from build123d import *

# Parameters (mm, degrees)
SKETCH1_W           = 31.5
SKETCH1_H           = 26
BOSS_EXTRUDE1_DEPTH = 33
SKETCH8_W           = 16
SKETCH8_H           = 20
BOSS_EXTRUDE2_DEPTH = 8
CUT_EXTRUDE1_START  = 10
CUT_EXTRUDE1_DEPTH  = 40.164116391
SKETCH3_R           = 2.85
CUT_EXTRUDE2_DEPTH  = 50.204293512
SKETCH6_R           = 6.25
CUT_EXTRUDE5_DEPTH  = 2
SKETCH4_R           = 2.35
CUT_EXTRUDE3_DEPTH  = 50.164116391
SKETCH5_R           = 6.5
CUT_EXTRUDE4_DEPTH  = 4
CHAMFER1_SIZE       = 3.5
CHAMFER3_SIZE       = 0.5
CHAMFER4_SIZE       = 12
CHAMFER5_SIZE       = 12
SKETCH10_R          = 4.428091906
BOSS_EXTRUDE4_DEPTH = 0.65
SKETCH11_R          = 4.527005536
SKETCH11_R_2        = 4.450513295
BOSS_EXTRUDE5_DEPTH = 0.65


with BuildPart() as part:
    # Sketch1 → Boss-Extrude1 (new body)
    with BuildSketch(Plane(origin=(0, 0, 0), x_dir=(1, 0, 0), z_dir=(0, 1, 0))):
        with Locations((0, -4.889880952)):
            Rectangle(SKETCH1_W, SKETCH1_H)
    extrude(amount=BOSS_EXTRUDE1_DEPTH)

    # Sketch8 → Boss-Extrude2 (add)
    with BuildSketch(Plane.XY.offset(17.889880952)):
        with Locations((23.75, 23)):
            Rectangle(SKETCH8_W, SKETCH8_H)
        with Locations((-23.75, 23)):
            Rectangle(SKETCH8_W, SKETCH8_H)
    extrude(amount=-BOSS_EXTRUDE2_DEPTH)

    # Sketch2 → Cut-Extrude1 (cut, through all)
    with BuildSketch(Plane.XZ.offset(-33).offset(CUT_EXTRUDE1_START)):
        Polygon((-11.25, 14.389880952), (-5.5, 14.389880952), (-5.5, 11.389880952), (5.5, 11.389880952), (5.5, 14.389880952), (11.25, 14.389880952), (11.25, -4.610119048), (5.5, -4.610119048), (5.5, -1.610119048), (-5.5, -1.610119048), (-5.5, -4.610119048), (-11.25, -4.610119048), align=None)
    extrude(amount=CUT_EXTRUDE1_DEPTH, mode=Mode.SUBTRACT)

    # Sketch3 → Cut-Extrude2 (cut, through all)
    with BuildSketch(Plane(origin=(0, 0, 9.889880952), x_dir=(-1, 0, 0), z_dir=(0, 0, -1))):
        with Locations((-23.75, 23)):
            Circle(SKETCH3_R)
        with Locations((23.75, 23)):
            Circle(SKETCH3_R)
    extrude(amount=-CUT_EXTRUDE2_DEPTH, mode=Mode.SUBTRACT)

    # Sketch6 → Cut-Extrude5 (cut)
    with BuildSketch(Plane(origin=(0, 0, 9.889880952), x_dir=(-1, 0, 0), z_dir=(0, 0, -1))):
        with Locations((-23.75, 23)):
            Circle(SKETCH6_R)
        with Locations((23.75, 23)):
            Circle(SKETCH6_R)
    extrude(amount=-CUT_EXTRUDE5_DEPTH, mode=Mode.SUBTRACT)

    # Sketch4 → Cut-Extrude3 (cut, through all)
    with BuildSketch(Plane(origin=(0, 33, 0), x_dir=(1, 0, 0), z_dir=(0, 1, 0))):
        with Locations(Location((0, -4.889880952, 0), (0, 0, 270))):
            Circle(SKETCH4_R)
    extrude(amount=-CUT_EXTRUDE3_DEPTH, mode=Mode.SUBTRACT)

    # Sketch5 → Cut-Extrude4 (cut)
    with BuildSketch(Plane(origin=(0, 33, 0), x_dir=(1, 0, 0), z_dir=(0, 1, 0))):
        with Locations(Location((0, -4.889880952, 0), (0, 0, 270))):
            Circle(SKETCH5_R)
    extrude(amount=-CUT_EXTRUDE4_DEPTH, mode=Mode.SUBTRACT)

    # Chamfer1
    chamfer1_edges = [part.edges().sort_by_distance(p)[0] for p in [
        (-15.75, 16.5, -8.110119048),
        (15.75, 16.5, -8.110119048),
    ]]
    chamfer(chamfer1_edges, length=CHAMFER1_SIZE)

    # Chamfer3
    chamfer3_edges = [part.edges().sort_by_distance(p)[0] for p in [
        (31.75, 23, 9.889880952),
        (-31.75, 23, 9.889880952),
    ]]
    chamfer(chamfer3_edges, length=CHAMFER3_SIZE)

    # Chamfer4
    # the kernel refuses this chamfer: 12 mm, written as the material it adds along each edge
    with BuildSketch(Plane(origin=(15.75, 13, 9.889880952), x_dir=(-0.027495876610586348, 0, -0.9996219169112968), z_dir=(0, 1, 0))) as chamfer4_piece_1_section:
        Polygon((CHAMFER4_SIZE * 0.999621916911, -CHAMFER4_SIZE * 0.0274958766106), (-CHAMFER4_SIZE * 0.0274958766106, -CHAMFER4_SIZE * 0.999621916911), (0, 0), align=None)
    chamfer4_piece_1 = extrude(amount=20, mode=Mode.PRIVATE)
    chamfer4_piece_1 = chamfer4_piece_1 - Plane(origin=(23.75, 23, -0.26462775), x_dir=(-1, 0, 0), z_dir=(0, 0, -1)) * Cylinder(6.25, 88, mode=Mode.PRIVATE)
    add(chamfer4_piece_1)
    with BuildSketch(Plane(origin=(-15.75, 13, 9.889880952), x_dir=(-0.9996219169112969, 0, 0.027495876610586348), z_dir=(0, 1, 0))) as chamfer4_piece_2_section:
        Polygon((CHAMFER4_SIZE * 0.999621916911, -CHAMFER4_SIZE * 0.0274958766106), (-CHAMFER4_SIZE * 0.0274958766106, -CHAMFER4_SIZE * 0.999621916911), (0, 0), align=None)
    chamfer4_piece_2 = extrude(amount=20, mode=Mode.PRIVATE)
    chamfer4_piece_2 = chamfer4_piece_2 - Plane(origin=(-23.75, 23, 8.187920604), x_dir=(-1, 0, 0), z_dir=(0, 0, -1)) * Cylinder(6.25, 88, mode=Mode.PRIVATE)
    add(chamfer4_piece_2)

    # Chamfer5
    chamfer5_edges = [part.edges().sort_by_distance(p)[0] for p in [
        (-15.75, 13, 7.889880952),
        (15.75, 13, 7.889880952),
    ]]
    chamfer(chamfer5_edges, length=CHAMFER5_SIZE)

    # Sketch10 → Boss-Extrude4 (add)
    with BuildSketch(Plane(origin=(0, 29, 0), x_dir=(1, 0, 0), z_dir=(0, 1, 0))):
        with Locations((0, -4.889880952)):
            Circle(SKETCH10_R)
    extrude(amount=-BOSS_EXTRUDE4_DEPTH)

    # Sketch11 → Boss-Extrude5 (add)
    with BuildSketch(Plane(origin=(0, 0, 11.889880952), x_dir=(-1, 0, 0), z_dir=(0, 0, -1))):
        with Locations((-23.75, 23)):
            Circle(SKETCH11_R)
        with Locations((23.75, 23)):
            Circle(SKETCH11_R_2)
    extrude(amount=-BOSS_EXTRUDE5_DEPTH)


solid = part.part
The model under review builds one solid part; all positions refer to its coordinate system, in mm. A direction names the side the tool comes from. Round coordinates to 2 decimals unless told otherwise and drop trailing zeros. Loops run counter-clockwise (first coordinate to the right, second up) from the corner with the lowest first, then second, coordinate; pieces in that order, holes last. Notation, with made-up numbers: (-30, 55.25) -> (20, 55.25) arc R15 ccw to (20, 63.25) -> close; hole circle Ø3 at (85, 63.5). An arc over 180 degrees is marked (long way). One line per question, with ' | ' between items. Start each with the question number.
Item 1: Wall thickness on line 1 along X through (y, z) = (4, -4.25); line 2 along Z through (x, y) = (-1.5, 6.5); line 3 along X through (y, z) = (12.5, 12.5): over which ranges is each line inside the solid? List them lowest first. Write a range as [from, to].
Item 2: Add section B-B, the plane y = 15.5. Write out the cut boundary in (x, z).
Item 3: Machinability: for faces 1 (the face through (-24, 23, 11.89)), 2 (the face through (0, 17, 17.89)), 3 (the face through (24, 23, 12.54)), 4 (the face through (-30, 13, 14)), 5 (the face through (8, 12, 14.39)), which of the approach directions +Z, -Z, +X, -X, +Y, -Y give a long, thin tool a straight path to every point of the face, cutting with its end or side? Answer none if there is none.
Item 4: Add section C-C, the plane x = 0. Write out the cut boundary in (y, z), then the cut area to 3 significant figures.
Item 5: Draft analysis for pull direction Y (two halves, no side actions). For faces 6 (the face through (0, 0, 13)), 7 (the face through (24, 23, 11.89)), 8 (the face through (-8, 12, 14.39)), state which applies: +Y half, -Y half, draft (parallel to the pull), parting line (faces both ways), or undercut.
Item 6: Add section D-D, the plane z = -3.5. Write out the cut boundary in (x, y), then the cut area to 3 significant figures.
Item 7: Add section A-A, the plane z = 13.75. Write out the cut boundary in (x, y), then the cut area to 3 significant figures.
Item 8: For pin 1 (14 mm diameter, centred on x = -24, y = 22.5, fed in from -Z); pin 2 (1.8 mm diameter, centred on x = -30, y = 23.5, fed in from -Z); pin 3 (9.5 mm diameter, centred on y = 12, z = 0, fed in from +X), all flat-tipped, find the tip position at first contact; note any pin that passes through.
Return value:
1) line 1: x = [-15.75, -11.25], [-5.5, 5.5], [11.25, 15.75] | line 2: z = [-8.11, -1.61], [11.39, 17.89] | line 3: x = [-27.25, -11.25], [-5.5, 5.5], [11.25, 27.25]
2) outline: (-31.75, 10.39) -> (-31.25, 9.89) -> (-27.75, 9.89) -> (-15.75, -2.11) -> (-15.75, -4.61) -> (-12.25, -8.11) -> (12.25, -8.11) -> (15.75, -4.61) -> (15.75, -2.11) -> (27.75, 9.89) -> (31.25, 9.89) -> (31.75, 10.39) -> (31.75, 17.89) -> (-31.75, 17.89) -> close; hole (-11.25, -4.61) -> (-5.5, -4.61) -> (-5.5, -1.61) -> (5.5, -1.61) -> (5.5, -4.61) -> (11.25, -4.61) -> (11.25, 14.39) -> (5.5, 14.39) -> (5.5, 11.39) -> (-5.5, 11.39) -> (-5.5, 14.39) -> (-11.25, 14.39) -> close
3) face 1: -Z | face 2: +Z, +X, -X, +Y, -Y | face 3: +Z | face 4: +Z, -Z, -X, -Y | face 5: -Y
4) outline: (0, -8.11) -> (33, -8.11) -> (33, -1.61) -> (29, -1.61) -> (29, 11.39) -> (33, 11.39) -> (33, 17.89) -> (0, 17.89) -> (0, 11.39) -> (23, 11.39) -> (23, 7.24) -> (28.35, 7.24) -> (28.35, 2.54) -> (23, 2.54) -> (23, -1.61) -> (0, -1.61) -> close | area: 482 mm2
5) face 6: -Y half | face 7: undercut | face 8: draft
6) outline: (-15.75, 0) -> (-11.25, 0) -> (-11.25, 23) -> (-5.5, 23) -> (-5.5, 0) -> (5.5, 0) -> (5.5, 23) -> (11.25, 23) -> (11.25, 0) -> (15.75, 0) -> (15.75, 33) -> (-15.75, 33) -> close | area: 775 mm2
7) outline: (-31.75, 13) -> (-27.75, 13) -> (-15.75, 1) -> (-15.75, 0) -> (-11.25, 0) -> (-11.25, 23) -> (-5.5, 23) -> (-5.5, 0) -> (5.5, 0) -> (5.5, 23) -> (11.25, 23) -> (11.25, 0) -> (15.75, 0) -> (15.75, 1) -> (27.75, 13) -> (31.75, 13) -> (31.75, 33) -> (-31.75, 33) -> close; hole circle Ø5.7 at (-23.75, 23); hole circle Ø5.7 at (23.75, 23) | area: 1,510 mm2
8) pin 1: stops at z = -0.86 | pin 2: stops at z = 9.89 | pin 3: stops at x = 22.61
